Geometry: final body of the model. Coordinates: model frame, mm. Give positions to 0.01 mm unless a question says otherwise; leave off trailing zeros. Write each loop counter-clockwise with the first axis right and the second up, starting at its lowest first coordinate (ties: lowest second). Pieces come first, ordered by that corner, then holes.
```python
from build123d import *

# Parameters (mm, degrees)
SKETCH1_R           = 13.75
SKETCH1_R_2         = 9.75
BOSS_EXTRUDE1_DEPTH = 2
CHAMFER1_SIZE       = 2
FILLET1_R           = 1.75


with BuildPart() as part:
    # Sketch1 → Boss-Extrude1 (new body)
    with BuildSketch(Plane(origin=(0, 0, 0), x_dir=(1, 0, 0), z_dir=(0, 1, 0))):
        with Locations(Location((0, 0, 0), (0, 0, 270))):
            Circle(SKETCH1_R)
        with Locations(Location((0, 0, 0), (0, 0, 270))):
            Circle(SKETCH1_R_2, mode=Mode.SUBTRACT)
    extrude(amount=BOSS_EXTRUDE1_DEPTH)

    # Chamfer1
    chamfer1_edges = [part.edges().sort_by_distance(p)[0] for p in [
        (0, 2, -13.75),
    ]]
    chamfer(chamfer1_edges, length=CHAMFER1_SIZE - 0.0001)  # a hair under: the kernel refuses the full size

    # Fillet1
    fillet1_edges = [part.edges().sort_by_distance(p)[0] for p in [
        (0, 0, -9.75),
    ]]
    fillet(fillet1_edges, radius=FILLET1_R)


solid = part.part
```
Item 1: Line query: L1, parallel to X at y = 1.95, z = 0; L2, parallel to X at y = 1.15, z = -8.25; L3, parallel to Z at x = 0.5, y = 1.5. Output: solid intervals per line, ascending.
Found:
L1: x = -11.8 to -9.75, 9.75 to 11.8
L2: x = -9.52 to -5.39, 5.39 to 9.52
L3: z = -12.24 to -9.76, 9.76 to 12.24
Item 2: Section C-C, the plane y = 1.4. Return the cut outline in (x, z).
Found:
outline: circle Ø24.7 at (0, 0); hole circle Ø19.57 at (0, 0)
Item 3: Pin query (flat end, axial travel): pin 1 Ø15.5 at (x, z) = (0, 0) entering from +Y. Return the tip coordinate at first contact, or that it passes through.
Found:
pin 1: passes through
